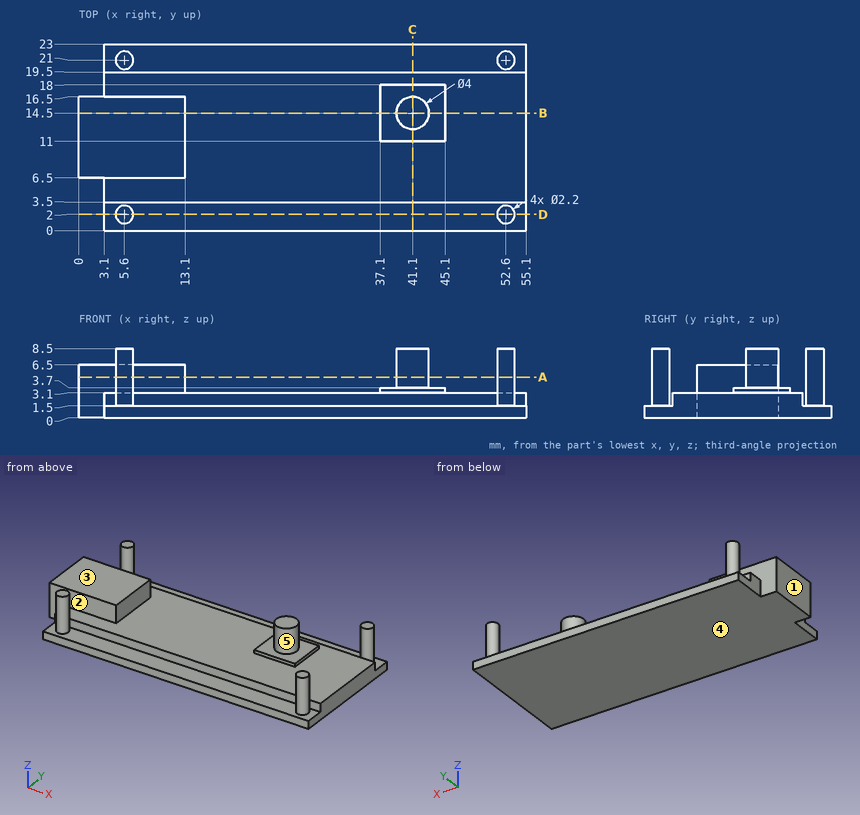
Part print with two shaded views. Sizes in mm from the minimum x, y, z corner. A direction names the side the tool comes from. Coordinates: 2 decimals unless noted, no trailing zeros. Order: outer loops, then holes, each group sorted by start corner. A loop starts at its lowest first (then second) coordinate and runs counter-clockwise, first axis right, second up. Notation, with made-up numbers: M 56,74 L 93,74 A20 cw 93,90 Z; hole C -0.5,51 d1. An arc over 180 degrees is marked long. One line per question, with ' | ' between items. Start each with the question number.
1. Flat gauge pins, fed straight in: P1, Ø1, axis at y = 13, z = 5, coming from the +X side; P2, Ø0.7, axis at y = 14.5, z = 3.5, coming from the +X side; P3, Ø6, axis at x = 24.5, y = 9.5, coming from the +Z side; P4, Ø5, axis at y = 5, z = 5, coming from the +X side. Where does each tip first touch, or does it go through?
2. Cut at D-D (y = 2). Write the cut outline in (x, z).
3. Mould opens along Y. For the marked faces 3, 4 and 5 say: +Y half, -Y half, draft (parallel to the pull), parting line (faces both ways), or undercut.
4. Cut at B-B (y = 14.5). Write the cut outline in (x, z).
5. Tool access for the marked faces 1 and 2: list every direction of +Z, -Z, +X, -X, +Y, -Y with a clear straight run to the whole face (end or side of a thin tool).
6. Wall check: line 1 along Z through (x, y) = (46, 16); line 2 along Y through (x, z) = (30.5, 3); line 3 along X through (y, z) = (2.75, 1). Give the ranges that are in metal, low to high. Write a range as [from, to].
7. Cut at A-A (z = 5). Write the cut outline in (x, y), plus the area to 3 significant figures.
8. Cut at C-C (x = 41.1). Write the cut outline in (y, z).
The answers:
1) P1: stops at x = 42.83 | P2: stops at x = 45.1 | P3: stops at z = 3.1 | P4: stops at x = 55.1
2) outline: M 3.1,0 L 55.1,0 L 55.1,1.5 L 53.7,1.5 L 53.7,8.5 L 51.5,8.5 L 51.5,1.5 L 6.7,1.5 L 6.7,8.5 L 4.5,8.5 L 4.5,1.5 L 3.1,1.5 Z
3) face 3: undercut | face 4: draft | face 5: parting line
4) outline: M 0,0 L 55.1,0 L 55.1,3.1 L 45.1,3.1 L 45.1,3.7 L 43.1,3.7 L 43.1,8.5 L 39.1,8.5 L 39.1,3.7 L 37.1,3.7 L 37.1,3.1 L 13.1,3.1 L 13.1,6.5 L 0,6.5 Z
5) face 1: +Z, -Z, -X, +Y, -Y | face 2: +Z, -X
6) line 1: z = [0, 3.1] | line 2: y = [3.5, 19.5] | line 3: x = [3.1, 55.1]
7) outline: M 0,6.5 L 13.1,6.5 L 13.1,16.5 L 0,16.5 Z; C 5.6,2 d2.2; C 5.6,21 d2.2; C 41.1,14.5 d4; C 52.6,2 d2.2; C 52.6,21 d2.2 | area: 159 mm2
8) outline: M 0,0 L 23,0 L 23,1.5 L 19.5,1.5 L 19.5,3.1 L 18,3.1 L 18,3.7 L 16.5,3.7 L 16.5,8.5 L 12.5,8.5 L 12.5,3.7 L 11,3.7 L 11,3.1 L 3.5,3.1 L 3.5,1.5 L 0,1.5 Z
